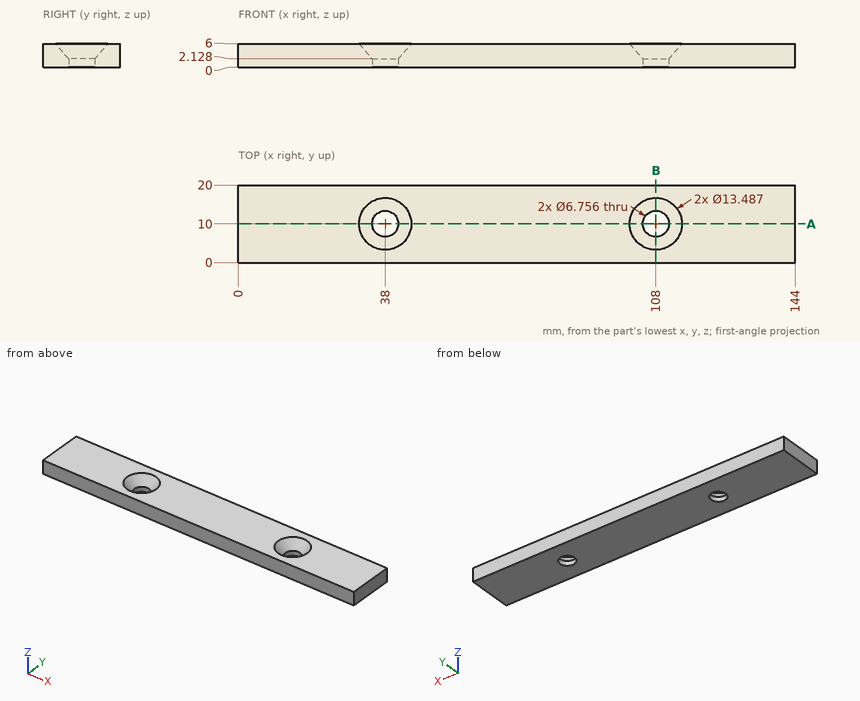
Geometry: see drawing. Coordinates: mm, zero at the bounding-box minimum. Give positions to 0.01 mm unless a question says otherwise; leave off trailing zeros. Order: outer loops, then holes, each group sorted by start corner. A loop starts at its lowest first (then second) coordinate and runs counter-clockwise, first axis right, second up. Notation, with made-up numbers: (6, -28) -> (52, -28) arc R17 ccw to (52, -20) -> close; hole circle Ø7 at (-18, -27). An arc over 180 degrees is marked (long way). Write each question's results on one line, items separated by ' | '. Start each with the question number.
1) Section A-A (y = 10). Return loops of the section in (x, z), then the cut area to 3 significant figures.
2) Line query: line 1 (X direction, y = 10, z = 1.5); line 2 (Y direction, x = 108, z = 0.7); line 3 (Y direction, x = 33, z = 5) (1 decimal). Output: solid intervals per line, ascending. Write a range as from..to.
3) Section B-B (x = 108). Return loops of the section in (y, z).
Calculated:
1) outline: (0, 0) -> (34.62, 0) -> (34.62, 2.13) -> (31.26, 6) -> (0, 6) -> close; (41.38, 0) -> (104.62, 0) -> (104.62, 2.13) -> (101.26, 6) -> (44.74, 6) -> (41.38, 2.13) -> close; (111.38, 0) -> (144, 0) -> (144, 6) -> (114.74, 6) -> (111.38, 2.13) -> close | area: 757 mm2
2) line 1: 0..34.62, 41.38..104.62, 111.38..144 | line 2: 0..6.62, 13.38..20 | line 3: 0..6.9, 13.1..20
3) outline: (0, 0) -> (6.62, 0) -> (6.62, 2.13) -> (3.26, 6) -> (0, 6) -> close; (13.38, 0) -> (20, 0) -> (20, 6) -> (16.74, 6) -> (13.38, 2.13) -> close
